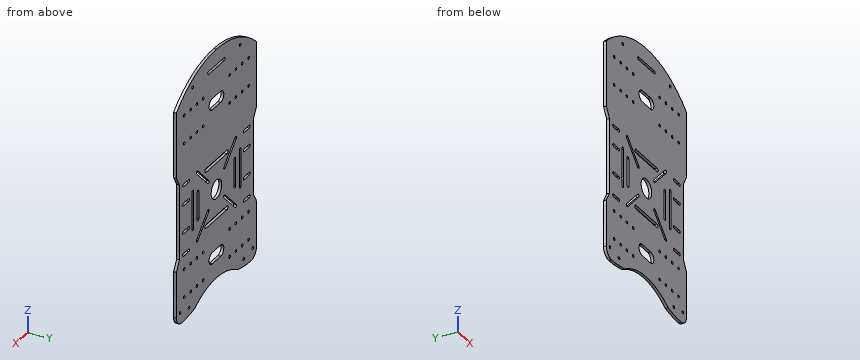
from build123d import *

# Parameters (mm, degrees)
SKETCH2_R           = 1.5
SKETCH2_R_2         = 10
BOSS_EXTRUDE1_DEPTH = 3


with BuildPart() as part:
    # Sketch2 → Boss-Extrude1 (new body)
    with BuildSketch(Plane(origin=(0, 0, 0), x_dir=(1, 0, 0), z_dir=(0, 1, 0))):
        with BuildLine():
            ThreePointArc((-41, 107), (-53.410321688, 109.247319267), (-66, 110))
            ThreePointArc((-66, 110), (-73.071067812, 107.071067812), (-76, 100))
            Line((-76, 100), (-76, 50.784609691))
            Line((-76, 50.784609691), (-70, 40.392304845))
            Line((-70, 40.392304845), (-70, -39.607695155))
            Line((-70, -39.607695155), (-76, -50))
            Line((-76, -50), (-76, -120))
            ThreePointArc((-76, -120), (-40.853396256, -142.228604363), (3.77e-07, -150))
            ThreePointArc((3.77e-07, -150), (40.853396607, -142.228604224), (76, -120))
            Line((76, -120), (76, -50))
            Line((76, -50), (70, -39.607695155))
            Line((70, -39.607695155), (70, 40.392304845))
            Line((70, 40.392304845), (76, 50.784609691))
            Line((76, 50.784609691), (76, 100))
            ThreePointArc((76, 100), (73.071067812, 107.071067812), (66, 110))
            ThreePointArc((66, 110), (53.410321688, 109.247319267), (41, 107))
            ThreePointArc((41, 107), (0, 95), (-41, 107))
        make_face()
        with Locations((-45, -132)):
            Circle(SKETCH2_R, mode=Mode.SUBTRACT)
        with Locations((-61, -110)):
            Circle(SKETCH2_R, mode=Mode.SUBTRACT)
        with Locations((-49, -110)):
            Circle(SKETCH2_R, mode=Mode.SUBTRACT)
        with Locations((-37, -110)):
            Circle(SKETCH2_R, mode=Mode.SUBTRACT)
        with Locations((-25, -110)):
            Circle(SKETCH2_R, mode=Mode.SUBTRACT)
        with BuildLine():
            ThreePointArc((-8, -101), (-14, -95), (-8, -89))
            Line((-8, -89), (8, -89))
            ThreePointArc((8, -89), (14, -95), (8, -101))
            Line((8, -101), (-8, -101))
        make_face(mode=Mode.SUBTRACT)
        with Locations((-61, -80)):
            Circle(SKETCH2_R, mode=Mode.SUBTRACT)
        with Locations((-49, -80)):
            Circle(SKETCH2_R, mode=Mode.SUBTRACT)
        with BuildLine():
            ThreePointArc((-62.5, -37), (-64, -35.5), (-62.5, -34))
            Line((-62.5, -34), (-52.5, -34))
            ThreePointArc((-52.5, -34), (-51, -35.5), (-52.5, -37))
            Line((-52.5, -37), (-62.5, -37))
        make_face(mode=Mode.SUBTRACT)
        with Locations((-37, -80)):
            Circle(SKETCH2_R, mode=Mode.SUBTRACT)
        with Locations((-25, -80)):
            Circle(SKETCH2_R, mode=Mode.SUBTRACT)
        with BuildLine():
            Line((-14.33273811, -16.454058454), (-35.545941546, -37.66726189))
            ThreePointArc((-35.545941546, -37.66726189), (-37.66726189, -37.66726189), (-37.66726189, -35.545941546))
            Line((-37.66726189, -35.545941546), (-16.454058454, -14.33273811))
            ThreePointArc((-16.454058454, -14.33273811), (-14.33273811, -14.33273811), (-14.33273811, -16.454058454))
        make_face(mode=Mode.SUBTRACT)
        with BuildLine():
            Line((20, -32), (-20, -32))
            ThreePointArc((-20, -32), (-22, -30), (-20, -28))
            Line((-20, -28), (20, -28))
            ThreePointArc((20, -28), (22, -30), (20, -32))
        make_face(mode=Mode.SUBTRACT)
        with BuildLine():
            ThreePointArc((-15, -133.5), (-16.5, -132), (-15, -130.5))
            Line((-15, -130.5), (15, -130.5))
            ThreePointArc((15, -130.5), (16.5, -132), (15, -133.5))
            Line((15, -133.5), (-15, -133.5))
        make_face(mode=Mode.SUBTRACT)
        with Locations((25, -110)):
            Circle(SKETCH2_R, mode=Mode.SUBTRACT)
        with Locations((37, -110)):
            Circle(SKETCH2_R, mode=Mode.SUBTRACT)
        with Locations((45, -132)):
            Circle(SKETCH2_R, mode=Mode.SUBTRACT)
        with Locations((49, -110)):
            Circle(SKETCH2_R, mode=Mode.SUBTRACT)
        with Locations((61, -110)):
            Circle(SKETCH2_R, mode=Mode.SUBTRACT)
        with Locations((25, -80)):
            Circle(SKETCH2_R, mode=Mode.SUBTRACT)
        with Locations((37, -80)):
            Circle(SKETCH2_R, mode=Mode.SUBTRACT)
        with BuildLine():
            ThreePointArc((37.66726189, -35.545941546), (37.66726189, -37.66726189), (35.545941546, -37.66726189))
            Line((35.545941546, -37.66726189), (14.33273811, -16.454058454))
            ThreePointArc((14.33273811, -16.454058454), (14.33273811, -14.33273811), (16.454058454, -14.33273811))
            Line((16.454058454, -14.33273811), (37.66726189, -35.545941546))
        make_face(mode=Mode.SUBTRACT)
        with Locations((49, -80)):
            Circle(SKETCH2_R, mode=Mode.SUBTRACT)
        with Locations((61, -80)):
            Circle(SKETCH2_R, mode=Mode.SUBTRACT)
        with BuildLine():
            Line((52.5, -34), (62.5, -34))
            ThreePointArc((62.5, -34), (64, -35.5), (62.5, -37))
            Line((62.5, -37), (52.5, -37))
            ThreePointArc((52.5, -37), (51, -35.5), (52.5, -34))
        make_face(mode=Mode.SUBTRACT)
        with BuildLine():
            Line((-52.5, -16.5), (-62.5, -16.5))
            ThreePointArc((-62.5, -16.5), (-64, -15), (-62.5, -13.5))
            Line((-62.5, -13.5), (-52.5, -13.5))
            ThreePointArc((-52.5, -13.5), (-51, -15), (-52.5, -16.5))
        make_face(mode=Mode.SUBTRACT)
        with BuildLine():
            ThreePointArc((-43.5, -20), (-45, -21.5), (-46.5, -20))
            Line((-46.5, -20), (-46.5, 20))
            ThreePointArc((-46.5, 20), (-45, 21.5), (-43.5, 20))
            Line((-43.5, 20), (-43.5, -20))
        make_face(mode=Mode.SUBTRACT)
        with BuildLine():
            ThreePointArc((-62.5, 13.5), (-64, 15), (-62.5, 16.5))
            Line((-62.5, 16.5), (-52.5, 16.5))
            ThreePointArc((-52.5, 16.5), (-51, 15), (-52.5, 13.5))
            Line((-52.5, 13.5), (-62.5, 13.5))
        make_face(mode=Mode.SUBTRACT)
        with BuildLine():
            ThreePointArc((-62.5, 37.5), (-64, 39), (-62.5, 40.5))
            Line((-62.5, 40.5), (-52.5, 40.5))
            ThreePointArc((-52.5, 40.5), (-51, 39), (-52.5, 37.5))
            Line((-52.5, 37.5), (-62.5, 37.5))
        make_face(mode=Mode.SUBTRACT)
        with BuildLine():
            ThreePointArc((-33.5, -15), (-35, -16.5), (-36.5, -15))
            Line((-36.5, -15), (-36.5, 15))
            ThreePointArc((-36.5, 15), (-35, 16.5), (-33.5, 15))
            Line((-33.5, 15), (-33.5, -15))
        make_face(mode=Mode.SUBTRACT)
        with BuildLine():
            ThreePointArc((-37.66726189, 35.545941546), (-37.66726189, 37.66726189), (-35.545941546, 37.66726189))
            Line((-35.545941546, 37.66726189), (-14.33273811, 16.454058454))
            ThreePointArc((-14.33273811, 16.454058454), (-14.33273811, 14.33273811), (-16.454058454, 14.33273811))
            Line((-16.454058454, 14.33273811), (-37.66726189, 35.545941546))
        make_face(mode=Mode.SUBTRACT)
        with BuildLine():
            ThreePointArc((-20, 28), (-22, 30), (-20, 32))
            Line((-20, 32), (20, 32))
            ThreePointArc((20, 32), (22, 30), (20, 28))
            Line((20, 28), (-20, 28))
        make_face(mode=Mode.SUBTRACT)
        with Locations((-61, 55)):
            Circle(SKETCH2_R, mode=Mode.SUBTRACT)
        with Locations((-49, 55)):
            Circle(SKETCH2_R, mode=Mode.SUBTRACT)
        with Locations((-61, 85)):
            Circle(SKETCH2_R, mode=Mode.SUBTRACT)
        with Locations((-69, 98)):
            Circle(SKETCH2_R, mode=Mode.SUBTRACT)
        with Locations((-49, 85)):
            Circle(SKETCH2_R, mode=Mode.SUBTRACT)
        with Locations((-52, 101)):
            Circle(SKETCH2_R, mode=Mode.SUBTRACT)
        with Locations((-37, 55)):
            Circle(SKETCH2_R, mode=Mode.SUBTRACT)
        with Locations((-25, 55)):
            Circle(SKETCH2_R, mode=Mode.SUBTRACT)
        with BuildLine():
            ThreePointArc((-8, 64), (-14, 70), (-8, 76))
            Line((-8, 76), (8, 76))
            ThreePointArc((8, 76), (14, 70), (8, 64))
            Line((8, 64), (-8, 64))
        make_face(mode=Mode.SUBTRACT)
        with Locations((-37, 85)):
            Circle(SKETCH2_R, mode=Mode.SUBTRACT)
        with Locations((-25, 85)):
            Circle(SKETCH2_R, mode=Mode.SUBTRACT)
        Circle(SKETCH2_R_2, mode=Mode.SUBTRACT)
        with BuildLine():
            Line((36.5, 15), (36.5, -15))
            ThreePointArc((36.5, -15), (35, -16.5), (33.5, -15))
            Line((33.5, -15), (33.5, 15))
            ThreePointArc((33.5, 15), (35, 16.5), (36.5, 15))
        make_face(mode=Mode.SUBTRACT)
        with BuildLine():
            Line((14.33273811, 16.454058454), (35.545941546, 37.66726189))
            ThreePointArc((35.545941546, 37.66726189), (37.66726189, 37.66726189), (37.66726189, 35.545941546))
            Line((37.66726189, 35.545941546), (16.454058454, 14.33273811))
            ThreePointArc((16.454058454, 14.33273811), (14.33273811, 14.33273811), (14.33273811, 16.454058454))
        make_face(mode=Mode.SUBTRACT)
        with BuildLine():
            Line((46.5, 20), (46.5, -20))
            ThreePointArc((46.5, -20), (45, -21.5), (43.5, -20))
            Line((43.5, -20), (43.5, 20))
            ThreePointArc((43.5, 20), (45, 21.5), (46.5, 20))
        make_face(mode=Mode.SUBTRACT)
        with BuildLine():
            ThreePointArc((62.5, -13.5), (64, -15), (62.5, -16.5))
            Line((62.5, -16.5), (52.5, -16.5))
            ThreePointArc((52.5, -16.5), (51, -15), (52.5, -13.5))
            Line((52.5, -13.5), (62.5, -13.5))
        make_face(mode=Mode.SUBTRACT)
        with BuildLine():
            Line((52.5, 16.5), (62.5, 16.5))
            ThreePointArc((62.5, 16.5), (64, 15), (62.5, 13.5))
            Line((62.5, 13.5), (52.5, 13.5))
            ThreePointArc((52.5, 13.5), (51, 15), (52.5, 16.5))
        make_face(mode=Mode.SUBTRACT)
        with BuildLine():
            Line((52.5, 40.5), (62.5, 40.5))
            ThreePointArc((62.5, 40.5), (64, 39), (62.5, 37.5))
            Line((62.5, 37.5), (52.5, 37.5))
            ThreePointArc((52.5, 37.5), (51, 39), (52.5, 40.5))
        make_face(mode=Mode.SUBTRACT)
        with Locations((25, 55)):
            Circle(SKETCH2_R, mode=Mode.SUBTRACT)
        with Locations((37, 55)):
            Circle(SKETCH2_R, mode=Mode.SUBTRACT)
        with Locations((25, 85)):
            Circle(SKETCH2_R, mode=Mode.SUBTRACT)
        with Locations((37, 85)):
            Circle(SKETCH2_R, mode=Mode.SUBTRACT)
        with Locations((49, 55)):
            Circle(SKETCH2_R, mode=Mode.SUBTRACT)
        with Locations((61, 55)):
            Circle(SKETCH2_R, mode=Mode.SUBTRACT)
        with Locations((49, 85)):
            Circle(SKETCH2_R, mode=Mode.SUBTRACT)
        with Locations((52, 101)):
            Circle(SKETCH2_R, mode=Mode.SUBTRACT)
        with Locations((61, 85)):
            Circle(SKETCH2_R, mode=Mode.SUBTRACT)
        with Locations((69, 98)):
            Circle(SKETCH2_R, mode=Mode.SUBTRACT)
    extrude(amount=BOSS_EXTRUDE1_DEPTH)


solid = part.part
The model under review builds one solid part; all positions refer to its coordinate system, in mm. Give positions to 0.01 mm unless a question says otherwise; leave off trailing zeros. Loops run counter-clockwise (first coordinate to the right, second up) from the corner with the lowest first, then second, coordinate; pieces in that order, holes last. Notation, with made-up numbers: (-5, 65) -> (21, 65) arc R22 cw to (21, 74) -> close; hole circle Ø2 at (58.5, 88.5). An arc over 180 degrees is marked (long way). Answer as a JSON object with one key per item and string values. Group by question number.
Q1. Take a section at B-B (z = 24.5). Write out the cut boundary in (x, y), plus the area to 3 significant figures.
Q2. Wall thickness on line 1 along X through (y, z) = (0.85, 11.5); line 2 along X through (y, z) = (2.8, -1); line 3 along Z through (x, y) = (-21.5, 0.25): over which ranges is each line inside the solid? List them lowest first.
Q3. Take a section at A-A (x = -56.5). Write out the cut boundary in (y, z), plus the area to 3 significant figures.
Q4. Take a section at C-C (x = -31). Write out the cut boundary in (y, z), plus the area to 3 significant figures.
Q5. Take a section at D-D (y = 0.8). State how many separate pieces and enclosed holes the cut face has, plus the area to 3 significant figures.
Q6. Insertion check: pin 1 (1.5 mm diameter, centred on x = 58, y = 2, fed in from -Z); pin 2 (1.5 mm diameter, centred on y = 2, z = -1, fed in from -X); pin 3 (1.5 mm diameter, centred on y = 2, z = -20, fed in from +X). Each pin has a flat end and moves straight along its axis. Give the tip position at first contact, or say it passes through.
Answer below:
{
 "1": {"outline": "(-70, 0) -> (-26.62, 0) -> (-26.62, 3) -> (-70, 3) -> close; (-22.38, 0) -> (22.38, 0) -> (22.38, 3) -> (-22.38, 3) -> close; (26.62, 0) -> (70, 0) -> (70, 3) -> (26.62, 3) -> close", "area": "395 mm2"},
 "2": {"line 1": "x = -70 to -46.5, -43.5 to -36.5, -33.5 to 33.5, 36.5 to 43.5, 46.5 to 70", "line 2": "x = -70 to -46.5, -43.5 to -36.5, -33.5 to -9.95, 9.95 to 33.5, 36.5 to 43.5, 46.5 to 70", "line 3": "z = -98.1 to -31.32, -28.68 to -23.62, -19.38 to 19.38, 23.62 to 28.68, 31.32 to 147.9"},
 "3": {"outline": "(0, -109.57) -> (3, -109.57) -> (3, -40.5) -> (0, -40.5) -> close; (0, -37.5) -> (3, -37.5) -> (3, -16.5) -> (0, -16.5) -> close; (0, -13.5) -> (3, -13.5) -> (3, 13.5) -> (0, 13.5) -> close; (0, 16.5) -> (3, 16.5) -> (3, 34) -> (0, 34) -> close; (0, 37) -> (3, 37) -> (3, 134.59) -> (0, 134.59) -> close", "area": "696 mm2"},
 "4": {"outline": "(0, -101.61) -> (3, -101.61) -> (3, -33.12) -> (0, -33.12) -> close; (0, -28.88) -> (3, -28.88) -> (3, 28.88) -> (0, 28.88) -> close; (0, 33.12) -> (3, 33.12) -> (3, 145.59) -> (0, 145.59) -> close", "area": "716 mm2"},
 "5": {"separate pieces": "1", "enclosed holes": "60", "area": "33,200 mm2"},
 "6": {"pin 1": "stops at z = -109.75", "pin 2": "stops at x = -70", "pin 3": "stops at x = 70"}
}
